Check sheet for the modelled part. Datum: model origin and axes. Units: mm. A direction names the side the tool comes from. Coordinates: 2 decimals unless noted, no trailing zeros. Loops run counter-clockwise (first coordinate to the right, second up) from the corner with the lowest first, then second, coordinate; pieces in that order, holes last. Notation, with made-up numbers: (-24, -36) - (2, -36) arc R13 cw to (2, -31) - close; hole circle Ø2 at (9.25, 68.5). An arc over 180 degrees is marked (long way). Write each question's results on one line, items separated by ' | '. Start each with the question number.
1. Tool access check on faces 5 (the face through (-0.33, 39.283, -7.493)), 6 (the face through (16.663, 27.762, 4.873)), 7 (the face through (4.88, 33.19, -1.08)). Record the directions out of +Z, -Z, +X, -X, +Y, -Y that give a thin tool (end or side, any length) a straight path to the whole face; none if there is none.
2. Thickness scan on line 1 (Z direction, x = 0, y = 34); line 2 (X direction, y = 23.5, z = 0). Record the ranges inside material, lowest first. Write a range as [from, to].
3. Draft check along X on faces 1 (the face through (-19.334, 27.748, -2.539)), 2 (the face through (3.16, 24.14, 7.62)), 3 (the face through (-14, 30.227, 1)), 4 (the face through (2.44, 39.68, -0.54)). Enter one of: released by +X, released by -X, zero draft, split by the parting line, or undercut.
4. Gauge pin test, flat ends, axial feed: P1, Ø4, axis at x = -15.26, z = -4.81, coming from the +Y side; P2, Ø3, axis at y = 21.5, z = -1, coming from the -X side; P3, Ø4, axis at y = 36, z = -8.5, coming from the +X side. Record the tip position at first contact, or that the pin passes through.
5. Cross-section at B-B (y = 32.75). Record the cut outline in (x, z).
6. Cross-section at A-A (y = 20). Record the cut outline in (x, z), and give its area (3 significant figures).
```python
from build123d import *

# Parameters (mm, degrees)
FILLET1_R          = 1
FILLET2_R          = 1
SKETCH3_R          = 1.5
CUT_EXTRUDE1_DEPTH = 20


with BuildPart() as part:
    # Sketch2 → Revolve1 (revolve)
    with BuildSketch(Plane(origin=(0, 0, 0), x_dir=(0, 0, -1), z_dir=(1, 0, 0))):
        Polygon((-2.5, 43.227272727), (-2.5, 36.227272727), (-5, 36.227272727), (-5, 30.227272727), (-8.25, 30.227272727), (-8.25, 18.227272727), (-12.5, 18.227272727), (-12.5, 25.227272727), (-19.5, 25.227272727), (-19.5, 30.227272727), (-12.5, 30.227272727), (-12.5, 34.227272727), (-7.5, 34.227272727), (-7.5, 43.227272727), align=None)
    revolve(axis=Axis((0, 55.454545455, 0), (0, -1, 0)))

    # Fillet1
    fillet1_edges = [part.edges().sort_by_distance(p)[0] for p in [
        (0, 34.227272727, -7.5),
        (0, 30.227272727, -12.5),
    ]]
    fillet(fillet1_edges, radius=FILLET1_R)

    # Fillet2
    fillet2_edges = [part.edges().sort_by_distance(p)[0] for p in [
        (0, 30.227272727, -19.5),
        (0, 25.227272727, -19.5),
    ]]
    fillet(fillet2_edges, radius=FILLET2_R)

    # Sketch3 → Cut-Extrude1 (cut)
    with BuildSketch(Plane(origin=(0, 30.227272727, 0), x_dir=(1, 0, 0), z_dir=(0, 1, 0))):
        with Locations(Location((15.176066716, -5.068234312, 0), (0, 0, 270))):
            Circle(SKETCH3_R)
        with Locations(Location((-15.258311064, 4.814970764, 0), (0, 0, 270))):
            Circle(SKETCH3_R)
    extrude(amount=-CUT_EXTRUDE1_DEPTH, mode=Mode.SUBTRACT)


solid = part.part
```
Established:
1) face 5: +Y | face 6: +Y, -Y | face 7: -Y
2) line 1: [-12.5, -5], [5, 12.5] | line 2: [-12.5, -8.25], [8.25, 12.5]
3) face 1: split by the parting line | face 2: undercut | face 3: zero draft | face 4: undercut
4) P1: y = 30.23 | P2: x = -12.5 | P3: x = 9.94
5) outline: circle Ø25 at (0, 0); hole circle Ø10 at (0, 0)
6) outline: circle Ø25 at (0, 0); hole circle Ø16.5 at (0, 0) | area: 277 mm^2
